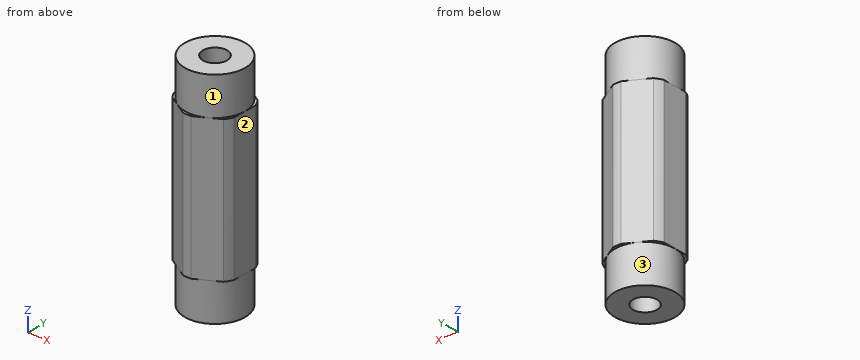
Autodesk Inventor part; units mm, degrees
ref_plane "YZ Plane" through (0, 0, 0) normal (1, 0, 0) x (0, 1, 0)
ref_plane "XZ Plane" through (0, 0, 0) normal (0, 1, 0) x (-1, 0, 0)
ref_plane "XY Plane" through (0, 0, 0) normal (0, 0, 1) x (1, 0, 0)
sketch "Sketch1" plane through (0, 0, 0) normal (0, 0, 1) x (1, 0, 0)
  line L0 (-6.35, -3.6662) -> (-6.35, 3.6662)
  line L1 (-6.35, 3.6662) -> (0, 7.3323)
  line L2 (0, 7.3323) -> (6.35, 3.6662)
  line L3 (6.35, 3.6662) -> (6.35, -3.6662)
  line L4 (6.35, -3.6662) -> (0, -7.3323)
  line L5 (0, -7.3323) -> (-6.35, -3.6662)
  point P0 (0, 0)
  point P1 (0, 0)
  dimension "Size" = 12.7
extrude "Extrusion1" add sketch "Sketch1" along normal mid plane 45.9994
sketch "Sketch3" plane through (0, 0, 22.9997) normal (0, 0, 1) x (1, 0, 0)
  line L0 (-6.35, 3.6662) -> (0, 7.3323) construction
  line L1 (0, 7.3323) -> (6.35, 3.6662) construction
  line L2 (6.35, 3.6662) -> (6.35, -3.6662) construction
  line L3 (6.35, -3.6662) -> (0, -7.3323) construction
  line L4 (0, -7.3323) -> (-6.35, -3.6662) construction
  line L5 (-6.35, -3.6662) -> (-6.35, 3.6662) construction
  point P0 (0, 0)
hole "Hole1" at (0, 0, 22.9997) direction (0, 0, -1) diameter 5.1054 end through all
sketch "Sketch4" plane through (0, 0, 22.9997) normal (0, 0, 1) x (1, 0, 0)
  circle A0 centre (0, 0) radius 2.5527 construction
  line L0 (-6.35, 3.6662) -> (0, 7.3323) construction
  line L1 (0, 7.3323) -> (6.35, 3.6662) construction
  line L2 (6.35, 3.6662) -> (6.35, -3.6662) construction
  line L3 (6.35, -3.6662) -> (0, -7.3323) construction
  line L4 (0, -7.3323) -> (-6.35, -3.6662) construction
  line L5 (-6.35, -3.6662) -> (-6.35, 3.6662) construction
  circle A1 centre (0, 0) radius 6.8771
  circle A2 centre (0, 0) radius 8.89
  dimension "thunder" = 13.7541
  dimension "d16" = 17.78
extrude "Extrusion3" cut sketch "Sketch4" against normal through all
sketch "Sketch5" plane through (0, 0, 22.9997) normal (0, 0, 1) x (1, 0, 0)
  circle A0 centre (0, 0) radius 6.35
  arc A1 (5.4616, -4.1791) -> (6.35, -2.6403) centre (0, 0) ccw
  line L0 (6.35, -2.6403) -> (6.35, 2.6403)
  arc A2 (6.35, 2.6403) -> (5.4616, 4.1791) centre (0, 0) ccw
  line L1 (5.4616, 4.1791) -> (0.8884, 6.8194)
  arc A3 (0.8884, 6.8194) -> (-0.8884, 6.8194) centre (0, 0) ccw
  line L2 (-0.8884, 6.8194) -> (-5.4616, 4.1791)
  arc A4 (-5.4616, 4.1791) -> (-6.35, 2.6403) centre (0, 0) ccw
  line L3 (-6.35, 2.6403) -> (-6.35, -2.6403)
  arc A5 (-6.35, -2.6403) -> (-5.4616, -4.1791) centre (0, 0) ccw
  line L4 (-5.4616, -4.1791) -> (-0.8884, -6.8194)
  arc A6 (-0.8884, -6.8194) -> (0.8884, -6.8194) centre (0, 0) ccw
  line L5 (0.8884, -6.8194) -> (5.4616, -4.1791)
  circle A7 centre (0, 0) radius 2.5527
  point P0 (3.175, -5.4993)
  point P1 (-3.175, -5.4993)
  point P2 (-6.35, 0)
  point P3 (-3.175, 5.4993)
  point P4 (3.175, 5.4993)
  point P5 (6.35, 0)
  dimension "d19" = 12.7
extrude "Extrusion4" cut sketch "Sketch5" against normal blind 8.001 contours L0 A1 L5 A0 | A0 L1 A2 L0 | A0 L2 A3 L1 | L5 A6 L4 A0 | A0 L3 A4 L2 | L4 A5 L3 A0
mirror "Mirror2" about plane through (0, 0, 0) normal (0, 0, 1) of "Extrusion4"
ref_plane "Work Plane1" through (0, 0, 0) normal (0, 0, 1) x (1, 0, 0)
equation "\"bearing\" = 25.4"
properties part number "GP5-029" material "Aluminum 6061"
The listing builds one solid part. Answer for the finished solid, in the listing's coordinates (mm). Face numbers are marked on the shaded views. A direction names the side the tool comes from. Give positions to 0.01 mm unless a question says otherwise; leave off trailing zeros. Order: outer loops, then holes, each group sorted by start corner. A loop starts at its lowest first (then second) coordinate and runs counter-clockwise, first axis right, second up. Notation, with made-up numbers: (-16, 85.25) -> (-2, 85.25) arc R24 cw to (-2, 97.25) -> close; hole circle Ø10 at (48, 86.25). An arc over 180 degrees is marked (long way). Answer as a JSON object with one key per item and string values. Group by question number.
Item 1: The part is cut by section D-D on y = -5. Write down the section's boundary in (x, z), and give its area (3 significant figures).
Item 2: A tool of negligible diameter and unlimited length cuts with its end or side. For the marked faces 1, 2 and 3, from which of +Z, -Z, +X, -X, +Y, -Y can it reach the whole face along a straight path? Write none if from no direction.
Item 3: Consider L1, parallel to Y at x = 0, z = 5; L2, parallel to X at y = 0, z = -12; L3, parallel to Z at x = -5.5, y = -4. Determine where each line is inside the solid, lowest interval first. Write a range as from..to.
Item 4: Flat-ended cylindrical pins translate along their axes: pin 1 (1.5 mm diameter, centred on y = -1.5, z = 16, fed in from +X); pin 2 (3 mm diameter, centred on x = 2.5, z = -6, fed in from +Y); pin 3 (1.5 mm diameter, centred on x = -5, z = 8.5, fed in from -Y). Find the tip coordinate at first contact, or state that the pin passes through.
Item 5: The part is cut by section B-B on y = -0.75. Write down the section's boundary in (x, z).
Item 6: The part is cut by section A-A on x = 0. Write down the section's boundary in (y, z), and give its area (3 significant figures).
Item 7: The part is cut by section C-C on z = -11.5. Write down the section's boundary in (x, y).
Result set:
{
 "1": {"outline": "(-4.04, -15) -> (-3.91, -15) -> (-3.91, -23) -> (3.91, -23) -> (3.91, -15) -> (4.04, -15) -> (4.04, 15) -> (3.91, 15) -> (3.91, 23) -> (-3.91, 23) -> (-3.91, 15) -> (-4.04, 15) -> close", "area": "368 mm²"},
 "2": {"face 1": "+Z", "face 2": "+Z, -Z, +X, +Y, -Y", "face 3": "-Z"},
 "3": {"L1": "-6.88..-2.55, 2.55..6.88", "L2": "-6.35..-2.55, 2.55..6.35", "L3": "-15..15"},
 "4": {"pin 1": "x = 6.31", "pin 2": "y = 6.75", "pin 3": "y = -4.88"},
 "5": {"outline": "(-6.35, -15) -> (-6.31, -15) -> (-6.31, -23) -> (-2.44, -23) -> (-2.44, 23) -> (-6.31, 23) -> (-6.31, 15) -> (-6.35, 15) -> close; (2.44, -23) -> (6.31, -23) -> (6.31, -15) -> (6.35, -15) -> (6.35, 15) -> (6.31, 15) -> (6.31, 23) -> (2.44, 23) -> close"},
 "6": {"outline": "(-6.88, -15) -> (-6.35, -15) -> (-6.35, -23) -> (-2.55, -23) -> (-2.55, 23) -> (-6.35, 23) -> (-6.35, 15) -> (-6.88, 15) -> close; (2.55, -23) -> (6.35, -23) -> (6.35, -15) -> (6.88, -15) -> (6.88, 15) -> (6.35, 15) -> (6.35, 23) -> (2.55, 23) -> close", "area": "381 mm²"},
 "7": {"outline": "(-6.35, -2.64) arc R6.88 ccw to (-5.46, -4.18) -> (-0.89, -6.82) arc R6.88 ccw to (0.89, -6.82) -> (5.46, -4.18) arc R6.88 ccw to (6.35, -2.64) -> (6.35, 2.64) arc R6.88 ccw to (5.46, 4.18) -> (0.89, 6.82) arc R6.88 ccw to (-0.89, 6.82) -> (-5.46, 4.18) arc R6.88 ccw to (-6.35, 2.64) -> close; hole circle Ø5.11 at (0, 0)"}
}
